from build123d import *

# Parameters (mm, degrees)
BOSS_EXTRUDE3_DEPTH = 117
CUT_EXTRUDE4_DEPTH  = 115
BOSS_EXTRUDE4_DEPTH = 87
CUT_EXTRUDE5_DEPTH  = 40
CUT_EXTRUDE6_DEPTH  = 4


with BuildPart() as part:
    # Sketch1 → Boss-Extrude3 (new body)
    with BuildSketch(Plane.XY):
        with BuildLine():
            ThreePointArc((2, 5.123475383), (1.017567048, 5.405049242), (0, 5.5))
            Line((0, 5.5), (0, 4.5))
            ThreePointArc((0, 4.5), (3.181980515, 3.181980515), (4.5, 0))
            ThreePointArc((4.5, 0), (3.181980515, -3.181980515), (0, -4.5))
            Line((0, -4.5), (0, -5.5))
            ThreePointArc((0, -5.5), (3.889087297, -3.889087297), (5.5, 0))
            ThreePointArc((5.5, 0), (4.541475531, 3.102418411), (2, 5.123475383))
        make_face()
        with BuildLine():
            Line((0, 4.5), (0, 5.5))
            ThreePointArc((0, 5.5), (-1.017567048, 5.405049242), (-2, 5.123475383))
            ThreePointArc((-2, 5.123475383), (-5.405049242, -1.017567048), (0, -5.5))
            Line((0, -5.5), (0, -4.5))
            ThreePointArc((0, -4.5), (-4.5, 0), (0, 4.5))
        make_face()
        with BuildLine():
            ThreePointArc((4.5, 0), (3.181980515, 3.181980515), (0, 4.5))
            Line((0, 4.5), (0, -4.5))
            ThreePointArc((0, -4.5), (3.181980515, -3.181980515), (4.5, 0))
        make_face()
        with BuildLine():
            Line((0, -4.5), (0, 4.5))
            ThreePointArc((0, 4.5), (-4.5, 0), (0, -4.5))
        make_face()
    extrude(amount=BOSS_EXTRUDE3_DEPTH)

    # Sketch1_3 → Cut-Extrude4 (cut)
    with BuildSketch(Plane.XY):
        with BuildLine():
            ThreePointArc((4.5, 0), (3.181980515, 3.181980515), (0, 4.5))
            Line((0, 4.5), (0, -4.5))
            ThreePointArc((0, -4.5), (3.181980515, -3.181980515), (4.5, 0))
        make_face()
        with BuildLine():
            Line((0, -4.5), (0, 4.5))
            ThreePointArc((0, 4.5), (-4.5, 0), (0, -4.5))
        make_face()
    extrude(amount=CUT_EXTRUDE4_DEPTH, mode=Mode.SUBTRACT)

    # Sketch1_4 → Boss-Extrude4 (add)
    with BuildSketch(Plane.XY):
        with BuildLine():
            Line((0, 5.5), (0, 8.623475383))
            Line((0, 8.623475383), (-2, 8.623475383))
            Line((-2, 8.623475383), (-2, 5.123475383))
            ThreePointArc((-2, 5.123475383), (-1.017567048, 5.405049242), (0, 5.5))
        make_face()
        with BuildLine():
            Line((2, 8.623475383), (0, 8.623475383))
            Line((0, 8.623475383), (0, 5.5))
            ThreePointArc((0, 5.5), (1.017567048, 5.405049242), (2, 5.123475383))
            Line((2, 5.123475383), (2, 8.623475383))
        make_face()
    extrude(amount=BOSS_EXTRUDE4_DEPTH)

    # Sketch1_5 → Cut-Extrude5 (cut)
    with BuildSketch(Plane.XY):
        with BuildLine():
            Line((2, 8.623475383), (0, 8.623475383))
            Line((0, 8.623475383), (0, 5.5))
            ThreePointArc((0, 5.5), (1.017567048, 5.405049242), (2, 5.123475383))
            Line((2, 5.123475383), (2, 8.623475383))
        make_face()
        with BuildLine():
            Line((0, 5.5), (0, 8.623475383))
            Line((0, 8.623475383), (-2, 8.623475383))
            Line((-2, 8.623475383), (-2, 5.123475383))
            ThreePointArc((-2, 5.123475383), (-1.017567048, 5.405049242), (0, 5.5))
        make_face()
    extrude(amount=CUT_EXTRUDE5_DEPTH, mode=Mode.SUBTRACT)

    # Sketch11 → Cut-Extrude6 (cut)
    with BuildSketch(Plane(origin=(2, 0, 0), x_dir=(0, 0, -1), z_dir=(1, 0, 0))):
        Polygon((-84.5, 5.179641377), (-85, 5.179641377), (-85.5, 8.664491245), (-84.5, 8.664491245), (-83.5, 8.664491245), (-84, 5.179641377), align=None)
        Polygon((-72.5, 5.179641377), (-73, 5.179641377), (-73.5, 8.664491245), (-72.5, 8.664491245), (-71.5, 8.664491245), (-72, 5.179641377), align=None)
        Polygon((-51.5, 5.179641377), (-52, 5.179641377), (-52.5, 8.664491245), (-51.5, 8.664491245), (-50.5, 8.664491245), (-51, 5.179641377), align=None)
        Polygon((-45.5, 5.179641377), (-46, 5.179641377), (-46.5, 8.664491245), (-45.5, 8.664491245), (-44.5, 8.664491245), (-45, 5.179641377), align=None)
        Polygon((-39.5, 5.179641377), (-40, 5.179641377), (-40.5, 8.664491245), (-39.5, 8.664491245), (-38.5, 8.664491245), (-39, 5.179641377), align=None)
        Polygon((-80.5, 8.664491245), (-81, 5.179641377), (-81.5, 5.179641377), (-82, 5.179641377), (-82.5, 8.664491245), (-81.5, 8.664491245), align=None)
        Polygon((-79.5, 8.664491245), (-79, 5.179641377), (-78.5, 5.179641377), (-78, 5.179641377), (-77.5, 8.664491245), (-78.5, 8.664491245), align=None)
        Polygon((-74.5, 8.664491245), (-75, 5.179641377), (-75.5, 5.179641377), (-76, 5.179641377), (-76.5, 8.664491245), (-75.5, 8.664491245), align=None)
        Polygon((-70.5, 8.664491245), (-70, 5.179641377), (-69.5, 5.179641377), (-69, 5.179641377), (-68.5, 8.664491245), (-69.5, 8.664491245), align=None)
        Polygon((-65.5, 8.664491245), (-66, 5.179641377), (-66.5, 5.179641377), (-67, 5.179641377), (-67.5, 8.664491245), (-66.5, 8.664491245), align=None)
        Polygon((-62.5, 8.664491245), (-63, 5.179641377), (-63.5, 5.179641377), (-64, 5.179641377), (-64.5, 8.664491245), (-63.5, 8.664491245), align=None)
        Polygon((-61.5, 8.664491245), (-61, 5.179641377), (-60.5, 5.179641377), (-60, 5.179641377), (-59.5, 8.664491245), (-60.5, 8.664491245), align=None)
        Polygon((-58.5, 8.664491245), (-58, 5.179641377), (-57.5, 5.179641377), (-57, 5.179641377), (-56.5, 8.664491245), (-57.5, 8.664491245), align=None)
        Polygon((-53.5, 8.664491245), (-54, 5.179641377), (-54.5, 5.179641377), (-55, 5.179641377), (-55.5, 8.664491245), (-54.5, 8.664491245), align=None)
        Polygon((-49.5, 8.664491245), (-49, 5.179641377), (-48.5, 5.179641377), (-48, 5.179641377), (-47.5, 8.664491245), (-48.5, 8.664491245), align=None)
        Polygon((-41.5, 8.664491245), (-42, 5.179641377), (-42.5, 5.179641377), (-43, 5.179641377), (-43.5, 8.664491245), (-42.5, 8.664491245), align=None)
        Polygon((-86.5, 8.664491245), (-87, 5.179641377), (-87.5, 5.179641377), (-88, 5.179641377), (-88.5, 8.664491245), (-87.5, 8.664491245), align=None)
    extrude(amount=-CUT_EXTRUDE6_DEPTH, mode=Mode.SUBTRACT)


solid = part.part
Could you check a few things on this model? Use its own coordinates, in mm. A direction names the side the tool comes from. Round coordinates to 2 decimals unless told otherwise and drop trailing zeros. Loops run counter-clockwise (first coordinate to the right, second up) from the corner with the lowest first, then second, coordinate; pieces in that order, holes last. Notation, with made-up numbers: (23.25, 84) -> (54.25, 84) arc R31 cw to (54.25, 114) -> close; hole circle Ø5 at (25, 42). An arc over 180 degrees is marked (long way). Use CSV: the item, a comma, the result in double quotes.
(1) For faces 1 (the flat face through (0.03, 6.93, 71.75)), 2 (the flat face through (-2, 7, 53)), which set-ups out of +Z, -Z, +X, -X, +Y, -Y let a thin tool reach every point of the face, with its end or its side?
Return value:
face 1,"+X, -X, +Y"
face 2,"+Z, -Z, -X, +Y"
(2) If I drill on probe 1 along Z at (x, y) = (-2.25, -0.5); probe 2 along Y at (x, z) = (-0.5, 57.5); probe 3 along Y at (x, z) = (2, 107.5), over which ranges is the centre line in solid material (lowest first)? Write a range as [from, to].
Return value:
probe 1,"z = [115, 117]"
probe 2,"y = [-5.48, -4.47], [4.47, 5.18]"
probe 3,"y = [-5.12, -4.03], [4.03, 5.12]"
(3) Suppose I cut it at C-C on y = 1.25. Write out the boundary of the cut face in (x, z), plus the area to 3 significant figures.
Return value:
outline,"(-5.36, 0) -> (-4.32, 0) -> (-4.32, 115) -> (4.32, 115) -> (4.32, 0) -> (5.36, 0) -> (5.36, 117) -> (-5.36, 117) -> close"
area,"259 mm²"
(4) Suppose I cut it at B-B on x = 3.25. Write out the boundary of the cut face in (y, z).
Return value:
outline,"(-4.44, 0) -> (-3.11, 0) -> (-3.11, 115) -> (3.11, 115) -> (3.11, 0) -> (4.44, 0) -> (4.44, 117) -> (-4.44, 117) -> close"
(5) Suppose I cut it at A-A on z = 19.5. Write out the boundary of the cut face in (x, y).
Return value:
outline,"circle Ø11 at (0, 0); hole circle Ø9 at (0, 0)"
(6) If we mould it in two halves opening along Z, with no side actions, what happens to faces 3 (the flat face through (0.028, 6.877, 85.244)), 4 (the flat face through (2, 7, 53))? For each: +Z half, -Z half, draft (parallel to the pull), parting line (faces both ways), or undercut.
Return value:
face 3,"undercut"
face 4,"draft"
(7) Will these pins go through, and if not, where does the flat tip stop? pin 1 Ø1 at (y, z) = (5, 17.5) entering from +X; pin 2 Ø0.8 at (x, z) = (0.5, 81.5) entering from +Y; pin 3 Ø6 at (y, z) = (5.5, 58) entering from +X.
Return value:
pin 1,"stops at x = 3.16"
pin 2,"stops at y = 5.18"
pin 3,"stops at x = 4.9"
